Autodesk Inventor part; units mm, degrees
ref_plane "YZ Plane" through (0, 0, 0) normal (1, 0, 0) x (0, 1, 0)
ref_plane "XZ Plane" through (0, 0, 0) normal (0, 1, 0) x (-1, 0, 0)
ref_plane "XY Plane" through (0, 0, 0) normal (0, 0, 1) x (1, 0, 0)
sketch "Sketch1" plane through (0, 0, 0) normal (0, 0, 1) x (1, 0, 0)
  circle A0 centre (0, 0) radius 3.4
  arc A1 (-4.06, -17.0946) -> (-5.63, -15.5246) centre (-5.63, -17.0946) ccw
  line L0 (-5.63, -15.5246) -> (-8.715, -15.5246)
  arc A2 (-10.285, -13.9546) -> (-8.715, -15.5246) centre (-8.715, -13.9546) ccw
  line L1 (-10.285, -13.9546) -> (-10.285, -13.4925)
  arc A3 (-10.0624, -12.9551) -> (-10.285, -13.4925) centre (-9.525, -13.4925) ccw
  line L2 (-10.0624, -12.9551) -> (-6.2171, -9.1098)
  arc A4 (-2.7773, -7.685) -> (-6.2171, -9.1098) centre (-2.7773, -12.5496) ccw
  line L3 (-2.7773, -7.685) -> (2.7773, -7.685)
  arc A5 (6.2171, -9.1098) -> (2.7773, -7.685) centre (2.7773, -12.5496) ccw
  line L4 (6.2171, -9.1098) -> (10.0624, -12.9551)
  arc A6 (10.285, -13.4925) -> (10.0624, -12.9551) centre (9.525, -13.4925) ccw
  line L5 (10.285, -13.4925) -> (10.285, -13.9546)
  arc A7 (8.715, -15.5246) -> (10.285, -13.9546) centre (8.715, -13.9546) ccw
  line L6 (8.715, -15.5246) -> (5.63, -15.5246)
  arc A8 (5.63, -15.5246) -> (4.06, -17.0946) centre (5.63, -17.0946) ccw
  line L7 (4.06, -17.0946) -> (4.06, -18.43)
  arc A9 (4.06, -18.43) -> (5.63, -20) centre (5.63, -18.43) ccw
  line L8 (5.63, -20) -> (16.83, -20)
  arc A10 (16.83, -20) -> (20, -16.83) centre (16.83, -16.83) ccw
  line L9 (20, -16.83) -> (20, -5.63)
  arc A11 (20, -5.63) -> (18.43, -4.06) centre (18.43, -5.63) ccw
  line L10 (18.43, -4.06) -> (17.25, -4.06)
  arc A12 (17.25, -4.06) -> (15.68, -5.63) centre (17.25, -5.63) ccw
  line L11 (15.68, -5.63) -> (15.68, -8.7154)
  arc A13 (14.11, -10.2854) -> (15.68, -8.7154) centre (14.11, -8.7154) ccw
  line L12 (14.11, -10.2854) -> (13.6201, -10.2854)
  arc A14 (13.1637, -9.947) -> (13.6201, -10.2854) centre (13.8117, -9.55) ccw
  line L13 (13.1637, -9.947) -> (9.0762, -5.8595)
  arc A15 (7.685, -2.5008) -> (9.0762, -5.8595) centre (12.435, -2.5008) ccw
  line L14 (7.685, -2.5008) -> (7.685, 2.5008)
  arc A16 (9.0762, 5.8595) -> (7.685, 2.5008) centre (12.435, 2.5008) ccw
  line L15 (9.0762, 5.8595) -> (13.2795, 10.0628)
  arc A17 (13.8169, 10.2854) -> (13.2795, 10.0628) centre (13.8169, 9.5254) ccw
  line L16 (13.8169, 10.2854) -> (14.11, 10.2854)
  arc A18 (15.68, 8.7154) -> (14.11, 10.2854) centre (14.11, 8.7154) ccw
  line L17 (15.68, 8.7154) -> (15.68, 5.63)
  arc A19 (15.68, 5.63) -> (17.25, 4.06) centre (17.25, 5.63) ccw
  line L18 (17.25, 4.06) -> (18.43, 4.06)
  arc A20 (18.43, 4.06) -> (20, 5.63) centre (18.43, 5.63) ccw
  line L19 (20, 5.63) -> (20, 16.83)
  arc A21 (20, 16.83) -> (16.83, 20) centre (16.83, 16.83) ccw
  line L20 (16.83, 20) -> (5.63, 20)
  arc A22 (5.63, 20) -> (4.06, 18.43) centre (5.63, 18.43) ccw
  line L21 (4.06, 18.43) -> (4.06, 17.0946)
  arc A23 (4.06, 17.0946) -> (5.63, 15.5246) centre (5.63, 17.0946) ccw
  line L22 (5.63, 15.5246) -> (8.715, 15.5246)
  arc A24 (10.285, 13.9546) -> (8.715, 15.5246) centre (8.715, 13.9546) ccw
  line L23 (10.285, 13.9546) -> (10.285, 13.4925)
  arc A25 (10.0624, 12.9551) -> (10.285, 13.4925) centre (9.525, 13.4925) ccw
  line L24 (10.0624, 12.9551) -> (6.2171, 9.1098)
  arc A26 (2.7773, 7.685) -> (6.2171, 9.1098) centre (2.7773, 12.5496) ccw
  line L25 (2.7773, 7.685) -> (-2.7773, 7.685)
  arc A27 (-6.2171, 9.1098) -> (-2.7773, 7.685) centre (-2.7773, 12.5496) ccw
  line L26 (-6.2171, 9.1098) -> (-10.0624, 12.9551)
  arc A28 (-10.285, 13.4925) -> (-10.0624, 12.9551) centre (-9.525, 13.4925) ccw
  line L27 (-10.285, 13.4925) -> (-10.285, 13.9546)
  arc A29 (-8.715, 15.5246) -> (-10.285, 13.9546) centre (-8.715, 13.9546) ccw
  line L28 (-8.715, 15.5246) -> (-5.63, 15.5246)
  arc A30 (-5.63, 15.5246) -> (-4.06, 17.0946) centre (-5.63, 17.0946) ccw
  line L29 (-4.06, 17.0946) -> (-4.06, 18.43)
  arc A31 (-4.06, 18.43) -> (-5.63, 20) centre (-5.63, 18.43) ccw
  line L30 (-5.63, 20) -> (-16.83, 20)
  arc A32 (-16.83, 20) -> (-20, 16.83) centre (-16.83, 16.83) ccw
  line L31 (-20, 16.83) -> (-20, 5.573)
  arc A33 (-20, 5.573) -> (-18.43, 4.003) centre (-18.43, 5.573) ccw
  line L32 (-18.43, 4.003) -> (-17.25, 4.003)
  arc A34 (-17.25, 4.003) -> (-15.68, 5.573) centre (-17.25, 5.573) ccw
  line L33 (-15.68, 5.573) -> (-15.68, 8.4757)
  arc A35 (-14.0552, 10.0447) -> (-15.68, 8.4757) centre (-14.11, 8.4757) ccw
  line L34 (-14.0552, 10.0447) -> (-13.7199, 10.033)
  arc A36 (-13.0405, 9.8238) -> (-13.7199, 10.033) centre (-13.5779, 9.2864) ccw
  line L35 (-13.0405, 9.8238) -> (-9.0762, 5.8595)
  arc A37 (-7.685, 2.5008) -> (-9.0762, 5.8595) centre (-12.435, 2.5008) ccw
  line L36 (-7.685, 2.5008) -> (-7.685, -2.5008)
  arc A38 (-9.0762, -5.8595) -> (-7.685, -2.5008) centre (-12.435, -2.5008) ccw
  line L37 (-9.0762, -5.8595) -> (-13.2795, -10.0628)
  arc A39 (-13.8169, -10.2854) -> (-13.2795, -10.0628) centre (-13.8169, -9.5254) ccw
  line L38 (-13.8169, -10.2854) -> (-14.11, -10.2854)
  arc A40 (-15.68, -8.7154) -> (-14.11, -10.2854) centre (-14.11, -8.7154) ccw
  line L39 (-15.68, -8.7154) -> (-15.68, -5.7579)
  arc A41 (-15.68, -5.7579) -> (-17.25, -4.1204) centre (-17.2485, -5.6904) ccw
  line L40 (-17.25, -4.1204) -> (-18.43, -4.1204)
  arc A42 (-18.43, -4.1204) -> (-20, -5.7579) centre (-18.4315, -5.6904) ccw
  line L41 (-20, -5.7579) -> (-20, -17.0184)
  arc A43 (-20, -17.0184) -> (-16.6746, -20) centre (-16.8354, -16.8341) ccw
  line L42 (-16.6746, -20) -> (-5.63, -20)
  arc A44 (-5.63, -20) -> (-4.06, -18.43) centre (-5.63, -18.43) ccw
  line L43 (-4.06, -18.43) -> (-4.06, -17.0946)
extrude "Extrusion1" add sketch "Sketch1" against normal blind 100
properties part number "40-4040-BLACK-FB"
Build history of the part. All positions in model axes, mm. A direction names the side the tool comes from. Give positions to 0.01 mm unless a question says otherwise; leave off trailing zeros. Order: outer loops, then holes, each group sorted by start corner. A loop starts at its lowest first (then second) coordinate and runs counter-clockwise, first axis right, second up. Notation, with made-up numbers: M 25.5,72 L 49.5,72 A22 cw 49.5,90 Z; hole C 23,-36 d3. An arc over 180 degrees is marked long. Use one line per item in the form item = value.
Q1. Pull direction X, two halves, no side cores. Call faces 1 (the cylindrical face through (8.037, -4.294, -49.3)), 2 (the flat face through (-7.685, 0, -49)), 3 (the cylindrical face through (19.096, 19.047, -49.3)): released by +X, released by -X, zero draft, split by the parting line, or undercut.
Conclusion:
face_1 = undercut
face_2 = released by -X
face_3 = released by +X
Q2. Which spindle directions (+Z, -Z, +X, -X, +Y, -Y) get a long thin tool onto all of the face, cutting with end or side? Do faces 4 (the flat face through (7.685, 0, -49)), 5 (the flat face through (-11, 20, -49)), 6 (the flat face through (0, 7.685, -49)), 7 (the flat face through (-15.68, 7, -49)). Say none if no direction does.
Conclusion:
face_4 = +Z, -Z, +X
face_5 = +Z, -Z, +X, -X, +Y
face_6 = +Z, -Z, +Y
face_7 = +Z, -Z
Q3. Wall check: probe 1 along Y at (x, z) = (0, -67.5) (3 decimals); probe 2 along X at (y, z) = (7, -91.5); probe 3 along Y at (x, z) = (9.5, -38.5). Give the ranges that are in metal, low to high.
Conclusion:
probe_1 = -7.685 to -3.4, 3.4 to 7.685
probe_2 = -20 to -15.68, -10.22 to 10.22, 15.68 to 20
probe_3 = -20 to -15.31, -12.39 to -6.28, 6.28 to 12.39, 15.31 to 20
Q4. Pin check, flat tips, straight feed: P1, Ø9, axis at x = 9, z = -34, coming from the -Y side; P2, Ø2, axis at x = 0, z = -77.5, coming from the -Y side (3 decimals); P3, Ø1.5, axis at y = 0.5, z = -65.5, coming from the -X side (3 decimals); P4, Ø9, axis at x = 0, y = 0, coming from the -Z side. Stop position of each tip, or through.
Conclusion:
P1 = -20
P2 = -7.685
P3 = -7.685
P4 = -100
Q5. Slice it at A-A, the plane x = 0. Write the cut outline in (y, z) (3 decimals).
Conclusion:
outline = M -7.685,-100 L -3.4,-100 L -3.4,0 L -7.685,0 Z; M 3.4,-100 L 7.685,-100 L 7.685,0 L 3.4,0 Z
